CAD build for the part. Positions are in the model's coordinates, mm. Face numbers are marked on the shaded views. A direction names the side the tool comes from. Round coordinates to 2 decimals unless told otherwise and drop trailing zeros. Order: outer loops, then holes, each group sorted by start corner. A loop starts at its lowest first (then second) coordinate and runs counter-clockwise, first axis right, second up. Notation, with made-up numbers: M -9,81.25 L 44,81.25 A9 cw 44,94.25 Z; hole C -25.75,-31 d2. An arc over 180 degrees is marked long. Put each result on its own line as item: value.
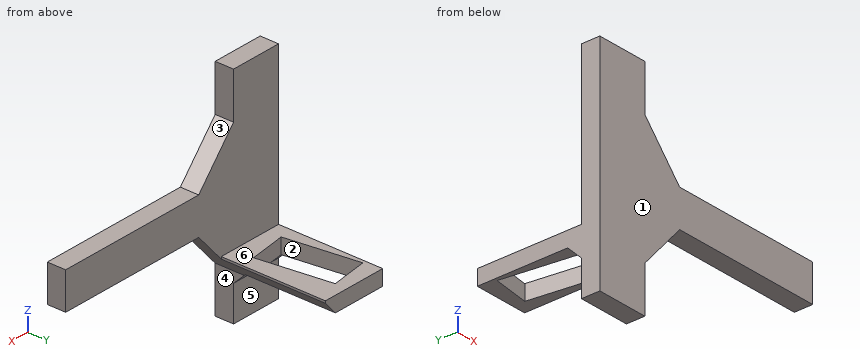
```python
from build123d import *

# Parameters (mm, degrees)
EXTRUDE_1_DEPTH     = 6
EXTRUDE_2_DEPTH     = 34
CUT_EXTRUDE_1_DEPTH = 5
CHAMFER_1_SIZE      = 4.5


with BuildPart() as part:
    # Эскиз1 → Бобышка-Вытянуть1 (new body)
    with BuildSketch(Plane(origin=(0, 0, 0), x_dir=(1, 0, 0), z_dir=(0, 1, 0))):
        Polygon((-49.854690153425345, 33.081252417759906), (-36.76089588655862, 18.081252417759906), (13.239104113441384, 18.08125241775991), (13.239104113441385, 6.081252417759905), (-36.76089588655862, 6.081252417759905), (-49.85469015342534, -8.918747582240094), (-49.85469015342534, -23.918747582240094), (-66.76089588655861, -23.918747582240094), (-66.76089588655861, 6.081252417759901), (-66.76089588655861, 18.081252417759902), (-66.76089588655861, 48.0812524177599), (-49.854690153425345, 48.0812524177599), align=None)
    extrude(amount=EXTRUDE_1_DEPTH)

    # Эскиз2 → Бобышка-Вытянуть2 (add)
    with BuildSketch(Plane(origin=(0, 6, 0), x_dir=(1, 0, 0), z_dir=(0, 1, 0))):
        Polygon((-66.76089588655861, 32.08125241775989), (-48.98177053563421, 32.08125241775989), (-45.2333870796828, 27.787176102421114), (-45.2333870796828, 27.081252417759895), (-66.76089588655861, 27.081252417759895), align=None)
    extrude(amount=EXTRUDE_2_DEPTH)

    # Эскиз3 → Вырез-Вытянуть1 (cut)
    with BuildSketch(Plane(origin=(0, 0, -32.08125241775989), x_dir=(-1, 0, 0), z_dir=(0, 0, -1))):
        Polygon((53.35223499298238, 36.15304870589925), (65.730585852252, 34.413384943898436), (62.39043142921044, 10.646951294100747), (50.012080569940814, 12.386615056101567), align=None)
    extrude(amount=-CUT_EXTRUDE_1_DEPTH, mode=Mode.SUBTRACT)

    # Фаска1
    chamfer_1_edges = [part.edges().sort_by_distance(p)[0] for p in [
        (-57.87133321109641, 6, -32.08125241775989),
    ]]
    chamfer(chamfer_1_edges, length=CHAMFER_1_SIZE)


solid = part.part
```
Item 1: Band-saw the part on A-A on y = 30.5. Give the cut face in (x, z).
Answers below:
outline: M -66.76,-32.08 L -65.18,-32.08 L -65.18,-27.08 L -66.76,-27.08 Z; M -52.56,-32.08 L -48.98,-32.08 L -45.23,-27.79 L -45.23,-27.08 L -52.56,-27.08 Z
Item 2: Mould opens along Y. For the marked faces 1, 2 and 3 say: pulls with the +Y half, pulls with the -Y half, needs draft (parallel to the pull), parting line crosses it, or undercut.
Answers below:
face 1: pulls with the -Y half
face 2: undercut
face 3: needs draft
Item 3: Band-saw the part on B-B on x = -55.5. Give the cut face in (y, z).
Answers below:
outline: M 0,-48.08 L 6,-48.08 L 6,-36.58 L 10.5,-32.08 L 11.62,-32.08 L 11.62,-27.08 L 6,-27.08 L 6,23.92 L 0,23.92 Z; M 35.85,-32.08 L 40,-32.08 L 40,-27.08 L 35.85,-27.08 Z
Item 4: Probe line 1 along Y through (x, z) = (-43, -19); line 2 along X through (y, z) = (6.5, -28.5); line 3 along Z through (x, y) = (-51, 8.5). List the from-to ranges inside material, lowest first. Write a range as [from, to].
Answers below:
line 1: [0, 6]
line 2: [-66.76, -45.86]
line 3: [-34.08, -27.08]
Item 5: Tool access for the marked faces 4, 5 and 6: list every direction of +Z, -Z, +X, -X, +Y, -Y with a clear straight run to the whole face (end or side of a thin tool).
Answers below:
face 4: -Z, +X, +Y, -Y
face 5: -Z, +X, -X, +Y
face 6: +Z, +X, -X, +Y
Item 6: Pin check, flat tips, straight feed: P1, Ø10, axis at x = -41.5, y = 30.5, coming from the +Z side; P2, Ø9, axis at x = -57, z = -41.5, coming from the +Y side; P3, Ø1.8, axis at y = 2.5, z = 17, coming from the +X side; P4, Ø5.5, axis at x = -59.5, y = 31, coming from the -Z side. Stop position of each tip, or through.
Answers below:
P1: z = -27.08
P2: y = 6
P3: x = -49.85
P4: through
Item 7: Band-saw the part on D-D on x = -11.5. Give the cut face in (y, z), and give its area (3 significant figures).
Answers below:
outline: M 0,-18.08 L 6,-18.08 L 6,-6.08 L 0,-6.08 Z
area: 72.0 mm²
Item 8: Band-saw the part on C-C on z = 15. Give the cut face in (x, y), and give its area (3 significant figures).
Answers below:
outline: M -66.76,0 L -49.85,0 L -49.85,6 L -66.76,6 Z
area: 101 mm²
